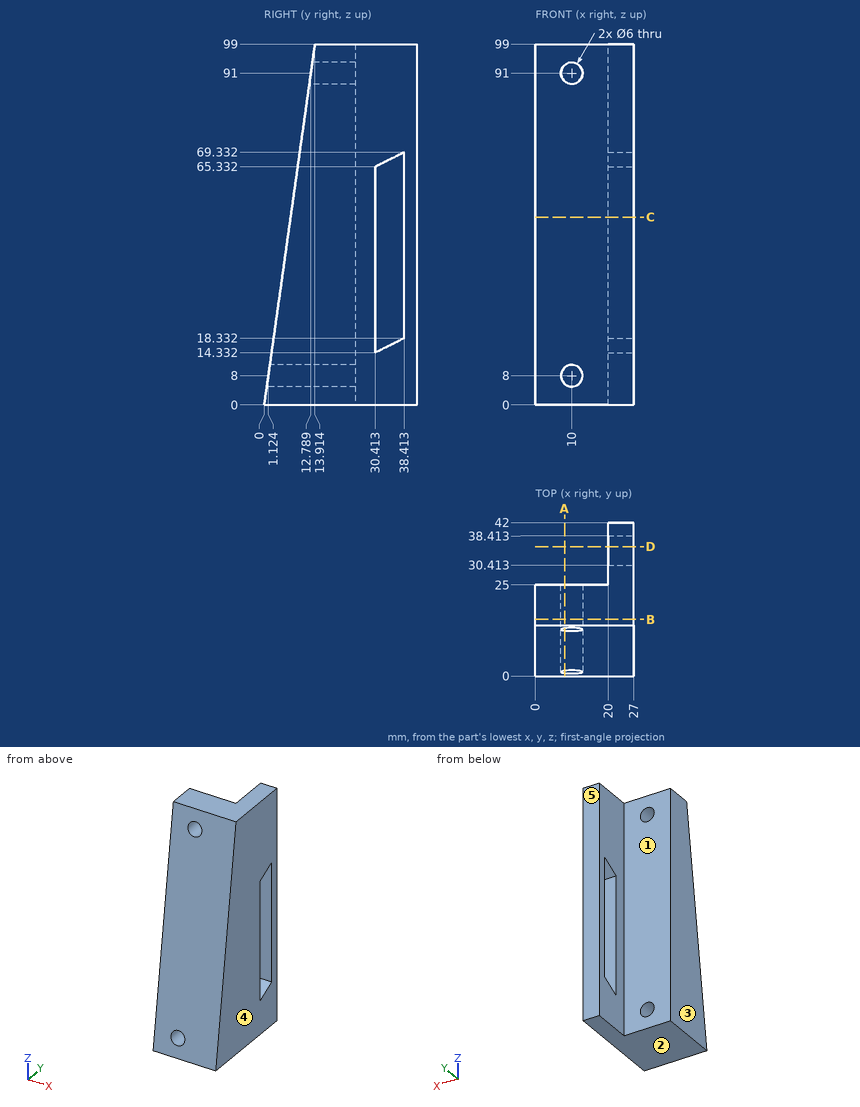
Can you work these out from the drawing? Everything is in mm from the part's minimum corner. A direction names the side the tool comes from. Round coordinates to 2 decimals unless told otherwise and drop trailing zeros. Loops run counter-clockwise (first coordinate to the right, second up) from the corner with the lowest first, then second, coordinate; pieces in that order, holes last. Notation, with made-up numbers: (16.25, 24) - (31.25, 24) arc R7 ccw to (31.25, 34) - close; hole circle Ø7 at (-16, -7.75). An arc over 180 degrees is marked (long way). Answer as CSV lines item,"result".
1. On a 3-axis mill with a long thin cutter (end or side, diameter ignored), from which of +Z, -Z, +X, -X, +Y, -Y can I reach the whole of each face in a straight line? I mean the marked faces 1 and 2. Say none if no direction works.
Filled in:
face 1,"+Z, -Z, -X, +Y"
face 2,"-Z, +X, -X, +Y, -Y"
2. For pin 1 Ø18.5 at (y, z) = (35, 26.5) entering from -X; pin 2 Ø3.5 at (x, z) = (23.5, 45) entering from -Y; pin 3 Ø9.5 at (x, z) = (10, 91) entering from -Y, each with a flat end and sliding along its axis, tell me the tip position at first contact or that it passes through.
Filled in:
pin 1,"stops at x = 20"
pin 2,"stops at y = 6.08"
pin 3,"stops at y = 12.12"
3. Please list where these lines run through material, in increasing order: line 1 along X through (y, z) = (9.5, 8); line 2 along Z through (x, y) = (10, 20); line 3 along Y through (x, z) = (22.25, 32). Write a range as [from, to].
Filled in:
line 1,"x = [0, 7], [13, 27]"
line 2,"z = [0, 5], [11, 88], [94, 99]"
line 3,"y = [4.5, 30.41], [38.41, 42]"
4. I want a section at B-B on y = 15.5. List the corners of the cut face in (x, z) for me, then the cut area to 3 significant figures.
Filled in:
outline,"(0, 0) - (27, 0) - (27, 99) - (0, 99) - close; hole circle Ø6 at (10, 8); hole circle Ø6 at (10, 91)"
area,"2,620 mm^2"
5. We'd pull the mould along X, two halves only. Please class the marked faces 3, 4 and 5: +X half, -X half, draft (parallel to the pull), parting line (faces both ways), or undercut.
Filled in:
face 3,"-X half"
face 4,"+X half"
face 5,"draft"
6. I want a section at C-C on z = 51.5. List the corners of the cut face in (x, y) for me.
Filled in:
outline,"(0, 7.24) - (27, 7.24) - (27, 30.41) - (20, 30.41) - (20, 25) - (0, 25) - close; (20, 38.41) - (27, 38.41) - (27, 42) - (20, 42) - close"
7. I want a section at A-A on x = 8. List the corners of the cut face in (y, z) for me (1 decimal), then the cut area to 4 significant figures.
Filled in:
outline,"(0, 0) - (25, 0) - (25, 5.8) - (0.8, 5.8) - close; (1.4, 10.2) - (25, 10.2) - (25, 88.8) - (12.5, 88.8) - close; (13.1, 93.2) - (25, 93.2) - (25, 99) - (13.9, 99) - close"
area,"1,625 mm^2"
8. I want a section at D-D on y = 35.5. List the corners of the cut face in (x, z) for me (1 decimal).
Filled in:
outline,"(20, 0) - (27, 0) - (27, 16.9) - (20, 16.9) - close; (20, 67.9) - (27, 67.9) - (27, 99) - (20, 99) - close"
